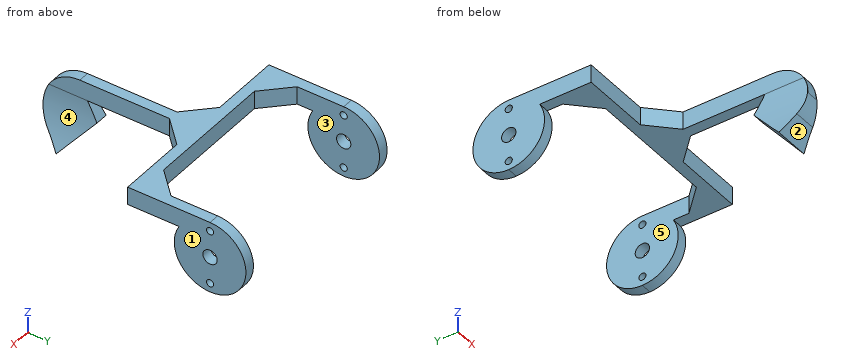
from build123d import *

# Parameters (mm, degrees)
BOSS_EXTRUDE1_DEPTH = 10
SKETCH2_OUTSIDE_W   = 35.602
SKETCH2_OUTSIDE_H   = 48.602
SKETCH2_OUTSIDE_R   = 2
CUT_EXTRUDE1_DEPTH  = 65.311741
SKETCH3_OUTSIDE_W   = 35.602
SKETCH3_OUTSIDE_H   = 48.602
CUT_EXTRUDE2_DEPTH  = 65.311741
BOSS_EXTRUDE2_DEPTH = 1.5
BOSS_EXTRUDE3_DEPTH = 5
SKETCH6_OUTSIDE_W   = 77.184
SKETCH6_OUTSIDE_H   = 42.134
CUT_EXTRUDE3_DEPTH  = 52.651745
SKETCH7_R           = 1
CUT_EXTRUDE4_DEPTH  = 73.669821
BOSS_EXTRUDE4_DEPTH = 5


with BuildPart() as part:
    # Sketch1 → Boss-Extrude1 (new, symmetric)
    with BuildSketch(Plane.XY):
        Polygon((0, 0), (-25, 0), (-25, 30), (-28, 30), (-28, -3), (0, -3), (28, -3), (28, 30), (25, 30), (25, 0), align=None)
    extrude(amount=BOSS_EXTRUDE1_DEPTH, both=True)

    # Sketch2 outside → Cut-Extrude1 (cut, through all)
    # profile 1 of 2: a face of its own
    with BuildSketch(Plane.ZY.offset(28)):
        with Locations((0, 13.5)):
            Rectangle(SKETCH2_OUTSIDE_W, SKETCH2_OUTSIDE_H)
        with BuildLine():
            Line((10, -3), (-10, -3))
            Line((-10, -3), (-10, 20))
            ThreePointArc((-10, 20), (0, 30), (10, 20))
            Line((10, 20), (10, -3))
        make_face(mode=Mode.SUBTRACT)
    # profile 2 of 2: a face of its own
    with BuildSketch(Plane.ZY.offset(28)):
        with Locations((0, 20)):
            Circle(SKETCH2_OUTSIDE_R)
    extrude(amount=-CUT_EXTRUDE1_DEPTH, mode=Mode.SUBTRACT)

    # Sketch3 outside → Cut-Extrude2 (cut, through all)
    with BuildSketch(Plane(origin=(28, 0, 0), x_dir=(0, 0, -1), z_dir=(1, 0, 0))):
        with Locations((0, 13.5)):
            Rectangle(SKETCH3_OUTSIDE_W, SKETCH3_OUTSIDE_H)
        with BuildLine():
            Line((-5, 11.339746), (-5, -3))
            Line((-5, -3), (-10, -3))
            Line((-10, -3), (-10, 20))
            ThreePointArc((-10, 20), (8.660254, 25), (-5, 11.339746))
        make_face(mode=Mode.SUBTRACT)
    extrude(amount=-CUT_EXTRUDE2_DEPTH, mode=Mode.SUBTRACT)

    # Sketch4 → Boss-Extrude2 (add, symmetric)
    with BuildSketch(Plane(origin=(0, 0, 0), x_dir=(0, 0, -1), z_dir=(1, 0, 0))):
        with BuildLine():
            Line((-10, -3), (-5, -3))
            Line((-5, -3), (-5, -32.886751))
            Line((-5, -32.886751), (0, -30))
            Line((0, -30), (0, -45))
            ThreePointArc((0, -45), (-7.071068, -42.071068), (-10, -35))
            Line((-10, -35), (-10, -3))
        make_face()
    extrude(amount=BOSS_EXTRUDE2_DEPTH, both=True)

    # Sketch5 → Boss-Extrude3 (add, symmetric)
    with BuildSketch(Plane(origin=(0, 0, 0), x_dir=(0, 0, -1), z_dir=(1, 0, 0))):
        with BuildLine():
            Line((0, -30), (-5, -32.886751))
            Line((-5, -32.886751), (-10, -32.886751))
            Line((-10, -32.886751), (-10, -35))
            ThreePointArc((-10, -35), (-4.414566, -43.972826), (6.102322, -42.922226))
            Line((6.102322, -42.922226), (10.950014, -39.188153))
            Line((10.950014, -39.188153), (0, -30))
        make_face()
    extrude(amount=BOSS_EXTRUDE3_DEPTH, both=True)

    # Sketch6 outside → Cut-Extrude3 (cut, through all)
    with BuildSketch(Plane.XZ.offset(3)):
        with Locations((0, -0.475)):
            Rectangle(SKETCH6_OUTSIDE_W, SKETCH6_OUTSIDE_H)
        with BuildLine():
            Line((-1.5, 10), (1.5, 10))
            Line((1.5, 10), (1.5, 5))
            ThreePointArc((1.5, 5), (2.385287, -3.164756), (5, -10.950014))
            Line((5, -10.950014), (-5, -10.950014))
            ThreePointArc((-5, -10.950014), (-2.385287, -3.164756), (-1.5, 5))
            Line((-1.5, 5), (-1.5, 10))
        make_face(mode=Mode.SUBTRACT)
    extrude(amount=CUT_EXTRUDE3_DEPTH, mode=Mode.SUBTRACT)

    # Sketch7 → Cut-Extrude4 (cut, through all)
    with BuildSketch(Plane(origin=(28, 0, 0), x_dir=(0, 0, -1), z_dir=(1, 0, 0))):
        with Locations((-7.5, 20)):
            Circle(SKETCH7_R)
        with Locations((7.5, 20)):
            Circle(SKETCH7_R)
    extrude(amount=-CUT_EXTRUDE4_DEPTH, mode=Mode.SUBTRACT)

    # Sketch8 → Boss-Extrude4 (add)
    with BuildSketch(Plane.XY.offset(10)):
        Polygon((-25, 0), (-25, 7), (-18, 0), align=None)
        Polygon((-8.5, -3), (-1.5, -3), (-1.5, -10), align=None)
        Polygon((1.5, -10), (1.5, -3), (8.5, -3), align=None)
        Polygon((18, 0), (25, 0), (25, 7), align=None)
    extrude(amount=-BOSS_EXTRUDE4_DEPTH)


solid = part.part
Here's how the part is built. I have some questions about the finished solid (model axes, mm). Face numbers are marked on the shaded views. A direction names the side the tool comes from. Round coordinates to 2 decimals unless told otherwise and drop trailing zeros. Write each loop counter-clockwise with the first axis right and the second up, starting at its lowest first coordinate (ties: lowest second). Pieces come first, ordered by that corner, then holes.
1. For the marked faces 4 and 5, which set-ups out of +Z, -Z, +X, -X, +Y, -Y let a thin tool reach every point of the face, with its end or its side?
2. If we mould it in two halves opening along X, with no side actions, what happens to the marked faces 1, 2 and 3? For each: released by +X, released by -X, zero draft, split by the parting line, or undercut.
3. Suppose I cut it at C-C (y = -13). List the corners of the cut face in (x, z) for me, and give its area (3 significant figures).
4. Suppose I cut it at A-A (z = -4.75). List the corners of the cut face in (x, y) for me, and give its area (3 significant figures).
5. I need wall thicknesses on L1, parallel to X at y = 25, z = 0.75; L2, parallel to Y at x = 27.3, z = 0; L3, parallel to Y at x = 11.5, z = 9. Which ranges of each line are inside material? Lowest first, please.
6. Suppose I cut it at B-B (x = 21). List the corners of the cut face in (y, z) for me, and give its area (3 significant figures).
7. Suppose I cut it at D-D (z = 7.5). List the corners of the cut face in (x, y) for me.
8. Will these pins go through, and if not, where does the flat tip stop? pin 1 Ø3 at (x, z) = (2, 7) entering from -Y; pin 2 Ø3.5 at (y, z) = (20, 0) entering from -X; pin 3 Ø4 at (x, z) = (6, 8) entering from +Y; pin 4 Ø4 at (x, z) = (17.5, 8.5) entering from -Y.
Answer sheet:
1. face 4: +Z, +X, +Y, -Y
1. face 5: +Z, -Z, +Y
2. face 1: released by +X
2. face 2: zero draft
2. face 3: undercut
3. outline: (-1.5, 5) - (1.5, 5) - (1.5, 10) - (-1.5, 10) - close
3. area: 15.0 mm2
4. outline: (-28, 11.2) - (-25, 11.2) - (-25, 28.8) - (-28, 28.8) - close; (-2.77, -43.8) - (2.77, -43.8) - (2.77, -33.99) - (-2.77, -33.99) - close; (25, 11.2) - (28, 11.2) - (28, 28.8) - (25, 28.8) - close
4. area: 160 mm2
5. L1: x = -28 to -25, 25 to 28
5. L2: y = 10 to 18, 22 to 30
5. L3: y = -3 to 0
6. outline: (-3, 5) - (3, 5) - (3, 10) - (-3, 10) - close
6. area: 30.0 mm2
7. outline: (-28, -3) - (-8.5, -3) - (-1.5, -10) - (-1.5, -41.61) - (1.5, -41.61) - (1.5, -10) - (8.5, -3) - (28, -3) - (28, 19) - (25, 19) - (25, 7) - (18, 0) - (-18, 0) - (-25, 7) - (-25, 19) - (-28, 19) - close; (-28, 21) - (-25, 21) - (-25, 26.61) - (-28, 26.61) - close; (25, 21) - (28, 21) - (28, 26.61) - (25, 26.61) - close
8. pin 1: stops at y = -43.29
8. pin 2: passes through
8. pin 3: stops at y = 0
8. pin 4: stops at y = -3
